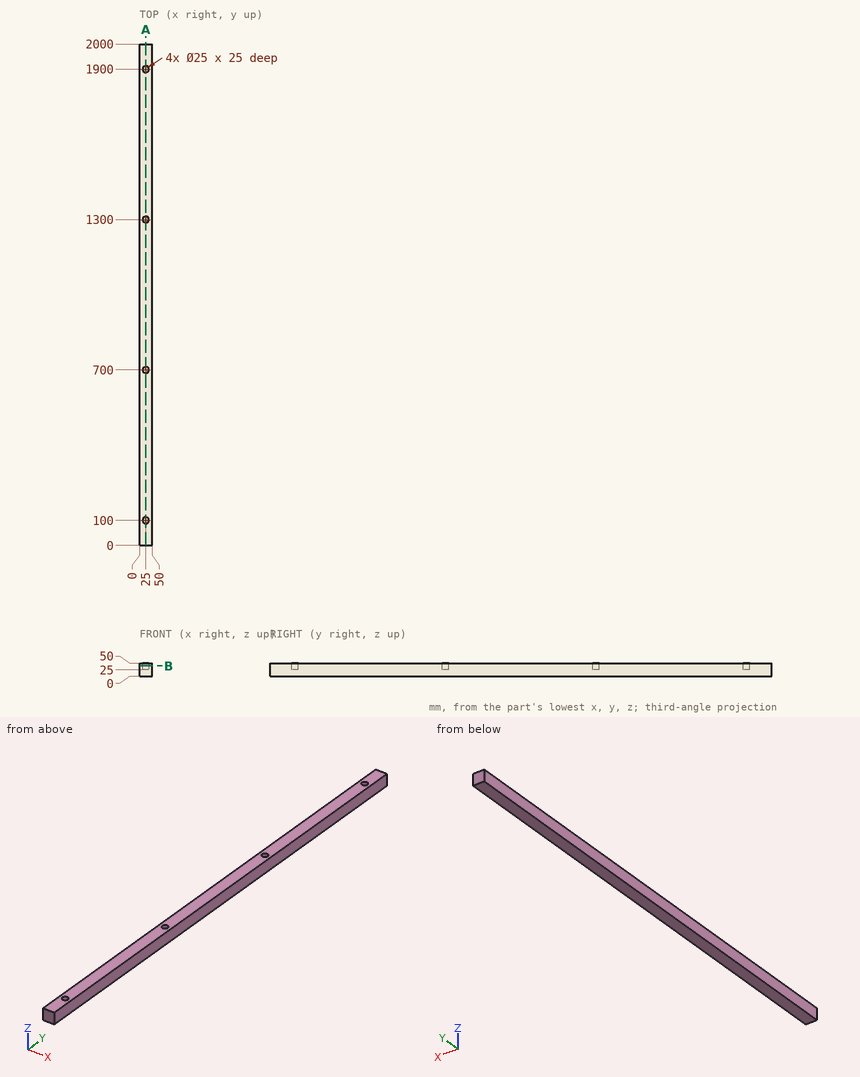
Can you work these out from the drawing? Everything is in mm from the part's minimum corner. Coordinates: 2 decimals unless noted, no trailing zeros. Loops run counter-clockwise (first coordinate to the right, second up) from the corner with the lowest first, then second, coordinate; pieces in that order, holes last. Notation, with made-up numbers: M 87.5,52 L 100.5,52 A12 cw 100.5,73 Z; hole C 41.25,77 d6. An arc over 180 degrees is marked long. One line per item, written item: value.
1. Will these pins go through, and if not, where does the flat tip stop? pin 1 Ø8 at (x, y) = (36.5, 312.5) entering from -Z; pin 2 Ø12.5 at (x, y) = (28.5, 700.5) entering from +Z.
Geometry says:
pin 1: stops at z = 0
pin 2: stops at z = 25
2. Please list where these lines run through material, in increasing order: probe 1 along Y at (x, z) = (25, 39); probe 2 along X at (y, z) = (1300, 40.5); probe 3 along Y at (x, z) = (29, 39).
Geometry says:
probe 1: y = 0 to 87.5, 112.5 to 687.5, 712.5 to 1287.5, 1312.5 to 1887.5, 1912.5 to 2000
probe 2: x = 0 to 12.5, 37.5 to 50
probe 3: y = 0 to 88.16, 111.84 to 688.16, 711.84 to 1288.16, 1311.84 to 1888.16, 1911.84 to 2000
3. Imagine slicing it at A-A (x = 25). List the corners of the cut face in (y, z) for me, and give its area (3 significant figures).
Geometry says:
outline: M 0,0 L 2000,0 L 2000,50 L 1912.5,50 L 1912.5,25 L 1887.5,25 L 1887.5,50 L 1312.5,50 L 1312.5,25 L 1287.5,25 L 1287.5,50 L 712.5,50 L 712.5,25 L 687.5,25 L 687.5,50 L 112.5,50 L 112.5,25 L 87.5,25 L 87.5,50 L 0,50 Z
area: 97,500 mm2
4. Imagine slicing it at B-B (z = 40). List the corners of the cut face in (x, y) for me, and give its area (3 significant figures).
Geometry says:
outline: M 0,0 L 50,0 L 50,2000 L 0,2000 Z; hole C 25,100 d25; hole C 25,700 d25; hole C 25,1300 d25; hole C 25,1900 d25
area: 98,000 mm2
